```python
from build123d import *

# Parameters (mm, degrees)
BOSS_EXTRUDE2_DEPTH = 30
SKETCH2_OUTSIDE_W   = 398.982
SKETCH2_OUTSIDE_H   = 1778.443
CUT_EXTRUDE3_DEPTH  = 1682.417983347


with BuildPart() as part:
    # Sketch1 → Boss-Extrude2 (new body)
    with BuildSketch(Plane(origin=(0, 0, 0), x_dir=(0, 0, -1), z_dir=(1, 0, 0))):
        with BuildLine():
            add(Edge.make_bspline(
                [(317.332343648, 655.186668482), (545.117144099, 641.097671469), (652.446570925, 854.768900431)],
                knots=[0.084059477, 0.084059477, 0.084059477, 1, 1, 1], degree=2))
            Line((317.332343648, 655.186668482), (1726.792532284, 506.936901497))
            Line((1726.792532284, 506.936901497), (1457.519541354, 1623.993731145))
            ThreePointArc((1457.519541354, 1623.993731145), (1431.012841469, 1665.338188153), (1384.60799847, 1681.417983247))
            Line((1384.60799847, 1681.417983247), (1050.440765915, 1681.417983247))
            ThreePointArc((1050.440765915, 1681.417983247), (1008.959277853, 1668.902270457), (981.322333542, 1635.532280531))
            Line((981.322333542, 1635.532280531), (652.446570925, 854.768900431))
        make_face()
    extrude(amount=BOSS_EXTRUDE2_DEPTH)

    # Sketch2 outside → Cut-Extrude3 (cut, through all)
    with BuildSketch(Plane(origin=(0, 0, 0), x_dir=(1, 0, 0), z_dir=(0, 1, 0))):
        with Locations((15, 1022.0625)):
            Rectangle(SKETCH2_OUTSIDE_W, SKETCH2_OUTSIDE_H)
        Polygon((15, 1726.792532284), (0, 317.332343643), (30, 317.332343643), align=None, mode=Mode.SUBTRACT)
    extrude(amount=CUT_EXTRUDE3_DEPTH, mode=Mode.SUBTRACT)


solid = part.part
```
The model under review builds one solid part; all positions refer to its coordinate system, in mm. Round coordinates to 2 decimals unless told otherwise and drop trailing zeros. Order: outer loops, then holes, each group sorted by start corner. A loop starts at its lowest first (then second) coordinate and runs counter-clockwise, first axis right, second up. Notation, with made-up numbers: M 58.5,-10.5 L 71.5,-10.5 A12 ccw 71.5,5.5 Z; hole C 78.25,86.5 d8. An arc over 180 degrees is marked long. Use a Markdown table: item, result.
1) Consider section B-B (z = -1191). Write out the cut boundary in (x, y).
Report:
| item | result |
|---|---|
| outline | M 9.3,563.29 L 20.7,563.29 L 20.7,1681.42 L 9.3,1681.42 Z |
2) Insertion check: pin 1 (5 mm diameter, centred on x = 21, z = -662.5, fed in from -Y); pin 2 (1.5 mm diameter, centred on x = 17.5, z = -662.5, fed in from -Y); pin 3 (2 mm diameter, centred on x = 22, y = 1024, fed in from +Z). Each pin has a flat end and moves straight along its axis. Give the tip position at first contact, or say it passes through.
Report:
| item | result |
|---|---|
| pin 1 | y = 618.62 |
| pin 2 | y = 618.8 |
| pin 3 | z = -723.31 |
3) Wall thickness on line 1 along X through (y, z) = (577.5, -1408.5); line 2 along X through (y, z) = (803.5, -1092); line 3 along Y through (x, z) = (25.5, -427.5): over which ranges is each line inside the solid? List them lowest first. Write a range as [from, to].
Report:
| item | result |
|---|---|
| line 1 | [11.61, 18.39] |
| line 2 | [8.24, 21.76] |
| line 3 | [643.6, 663.23] |
4) Consider section A-A (y = 1248). Write out the cut boundary in (x, z) (3 decimals).
Report:
| item | result |
|---|---|
| outline | M 5.329,-818.085 L 13.099,-1548.155 L 16.901,-1548.155 L 24.671,-818.085 Z |
